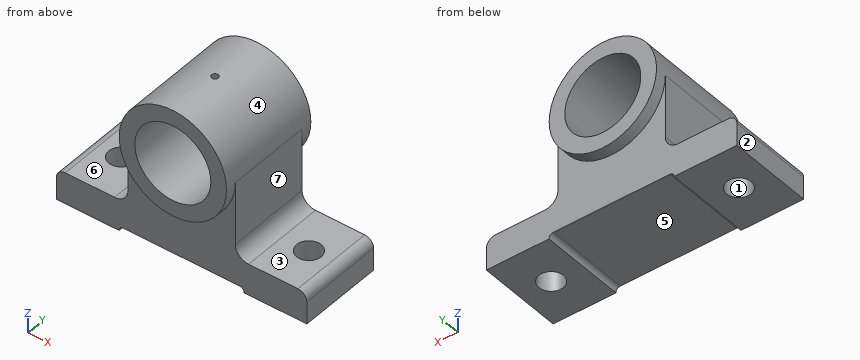
from build123d import *

# Parameters (mm, degrees)
F0_R     = 26.9875
F1_DEPTH = 38.1
F2_DEPTH = 30.1625
F3_R     = 8.73125
F4_DEPTH = 76.201
F5_R     = 2.38125
F6_DEPTH = 38.101
F7_R     = 9.525
F8_R     = 6.35
F9_R     = 3.17499


# Not quite as in the source:
# - a fillet or chamfer is up to 0.001 mm smaller than in the source, because OpenCascade refuses the exact size


with BuildPart() as f1:
    # F0 (on Front) → F1 (new body, symmetric)
    with BuildSketch(Plane.XZ):
        with BuildLine():
            ThreePointArc((-38.1, 0), (0, -38.1), (38.1, 0))
            ThreePointArc((38.1, 0), (0, 38.1), (-38.1, 0))
        make_face()
        Circle(F0_R, mode=Mode.SUBTRACT)
    extrude(amount=F1_DEPTH, both=True)

    # F0 (on Front) → F2 (join, symmetric)
    with BuildSketch(Plane.XZ):
        with BuildLine():
            ThreePointArc((-38.1, 0), (0, -38.1), (38.1, 0))
            ThreePointArc((38.1, 0), (0, 38.1), (-38.1, 0))
        make_face()
        Circle(F0_R, mode=Mode.SUBTRACT)
        with BuildLine():
            Line((38.1, -53.975), (38.1, 0))
            ThreePointArc((38.1, 0), (0, -38.1), (-38.1, 0))
            Line((-38.1, 0), (-38.1, -53.975))
            Line((-38.1, -53.975), (-88.9, -53.975))
            Line((-88.9, -53.975), (-88.9, -76.2))
            Line((-88.9, -76.2), (-44.45, -76.2))
            Line((-44.45, -76.2), (-44.45, -73.025))
            Line((-44.45, -73.025), (0, -73.025))
            Line((0, -73.025), (44.45, -73.025))
            Line((44.45, -73.025), (44.45, -76.2))
            Line((44.45, -76.2), (88.9, -76.2))
            Line((88.9, -76.2), (88.9, -53.975))
            Line((88.9, -53.975), (38.1, -53.975))
        make_face()
    extrude(amount=F2_DEPTH, both=True)

    # F3 (on Top) → F4 (cut, through all)
    with BuildSketch(Plane.XY):
        with Locations((-66.675, 0)):
            Circle(F3_R)
        with Locations((66.675, 0)):
            Circle(F3_R)
    extrude(amount=-F4_DEPTH, mode=Mode.SUBTRACT)

    # F5 (on Top) → F6 (cut, through all)
    with BuildSketch(Plane.XY):
        Circle(F5_R)
    extrude(amount=F6_DEPTH, mode=Mode.SUBTRACT)

    # F7
    f7_edges = [f1.edges().sort_by_distance(p)[0] for p in [
        (38.1, 0, -53.975),
        (-38.1, 0, -53.975),
    ]]
    fillet(f7_edges, radius=F7_R)

    # F8
    f8_edges = [f1.edges().sort_by_distance(p)[0] for p in [
        (-88.9, 0, -53.975),
        (88.9, 0, -53.975),
    ]]
    fillet(f8_edges, radius=F8_R)

    # F9 (radius 3.175 in the source; OpenCascade refuses exactly that, so slightly less here)
    f9_edges = [f1.edges().sort_by_distance(p)[0] for p in [
        (-44.45, 0, -73.025),
        (44.45, 0, -73.025),
    ]]
    fillet(f9_edges, radius=F9_R)


solid = f1.part
For this review, take the finished solid that the model builds, in its own axes (mm). Face numbers are marked on the shaded views. A direction names the side the tool comes from. Coordinates: 2 decimals unless noted, no trailing zeros. Order: outer loops, then holes, each group sorted by start corner. A loop starts at its lowest first (then second) coordinate and runs counter-clockwise, first axis right, second up. Notation, with made-up numbers: (-24.5, 18.25) - (-15.5, 18.25) arc R12 ccw to (-15.5, 29.25) - close; hole circle Ø9 at (51.5, 80). An arc over 180 degrees is marked (long way). Answer as CSV lines item,"result". Start each with the question number.
1) Insertion check: P1, Ø4, axis at y = 29, z = 23.5, coming from the +X side; P2, Ø12, axis at y = 22.5, z = -26.5, coming from the -X side; P3, Ø3, axis at y = 28, z = -49, coming from the +X side. Each pin has a flat end and moves straight along its axis. Give the tip position at first contact, or say it passes through.
2) To check wall thickness, follow line 1 along X through (y, z) = (-27.5, -1.5); line 2 along Z through (x, y) = (70.5, -16) (3 decimals); line 3 along X through (y, z) = (31, -19.5). State the ranges of each line that lie inside material, in increasing order. Write a range as [from, to].
3) Add section B-B (x = 0). State the section outline as (y, z) points (1 decimal), then the cut area to 3 significant figures.
4) Add section D-D (x = -60). State the section outline as (y, z) points (1 decimal).
5) Draft analysis for pull direction X (two halves, no side actions). For the marked faces 1, 2, 3 and 4, state which applies: +X half, -X half, draft (parallel to the pull), parting line (faces both ways), or undercut.
6) Add section C-C (z = 6.5). State the section outline as (x, y) points.
7) Machinability: for the marked faces 5, 6 and 7, which of the approach directions +Z, -Z, +X, -X, +Y, -Y give a long, thin tool a straight path to every point of the face, cutting with its end or side? Answer none if there is none.
Result:
1,P1,"x = 31.45"
1,P2,"x = -38.1"
1,P3,"x = 40.27"
2,line 1,"[-38.1, -26.95], [26.95, 38.1]"
2,line 2,"[-76.2, -53.975]"
2,line 3,"[-32.73, -18.66], [18.66, 32.73]"
3,outline,"(-38.1, -38.1) - (-30.2, -38.1) - (-30.2, -73) - (30.2, -73) - (30.2, -38.1) - (38.1, -38.1) - (38.1, -27) - (-38.1, -27) - close; (-38.1, 27) - (-2.4, 27) - (-2.4, 38.1) - (-38.1, 38.1) - close; (2.4, 27) - (38.1, 27) - (38.1, 38.1) - (2.4, 38.1) - close"
3,area,"3,750 mm^2"
4,outline,"(-30.2, -76.2) - (-5.6, -76.2) - (-5.6, -54) - (-30.2, -54) - close; (5.6, -76.2) - (30.2, -76.2) - (30.2, -54) - (5.6, -54) - close"
5,face 1,"undercut"
5,face 2,"-X half"
5,face 3,"draft"
5,face 4,"parting line"
6,outline,"(-37.54, -38.1) - (-26.19, -38.1) - (-26.19, 38.1) - (-37.54, 38.1) - close; (26.19, -38.1) - (37.54, -38.1) - (37.54, 38.1) - (26.19, 38.1) - close"
7,face 5,"-Z, +Y, -Y"
7,face 6,"+Z, -X, +Y, -Y"
7,face 7,"+Z, +X, +Y, -Y"
